Could you check a few things on this drawing? It's one solid part, dimensions in mm from its lowest x, y, z. Give positions to 0.01 mm unless a question says otherwise; leave off trailing zeros. Order: outer loops, then holes, each group sorted by start corner. A loop starts at its lowest first (then second) coordinate and runs counter-clockwise, first axis right, second up. Notation, with made-up numbers: (-7.5, 4.5) - (28.5, 4.5) arc R16 ccw to (28.5, 22.5) - close; hole circle Ø10 at (35, -30). An arc over 180 degrees is marked (long way). Return JSON: item names as keys, results as strings.
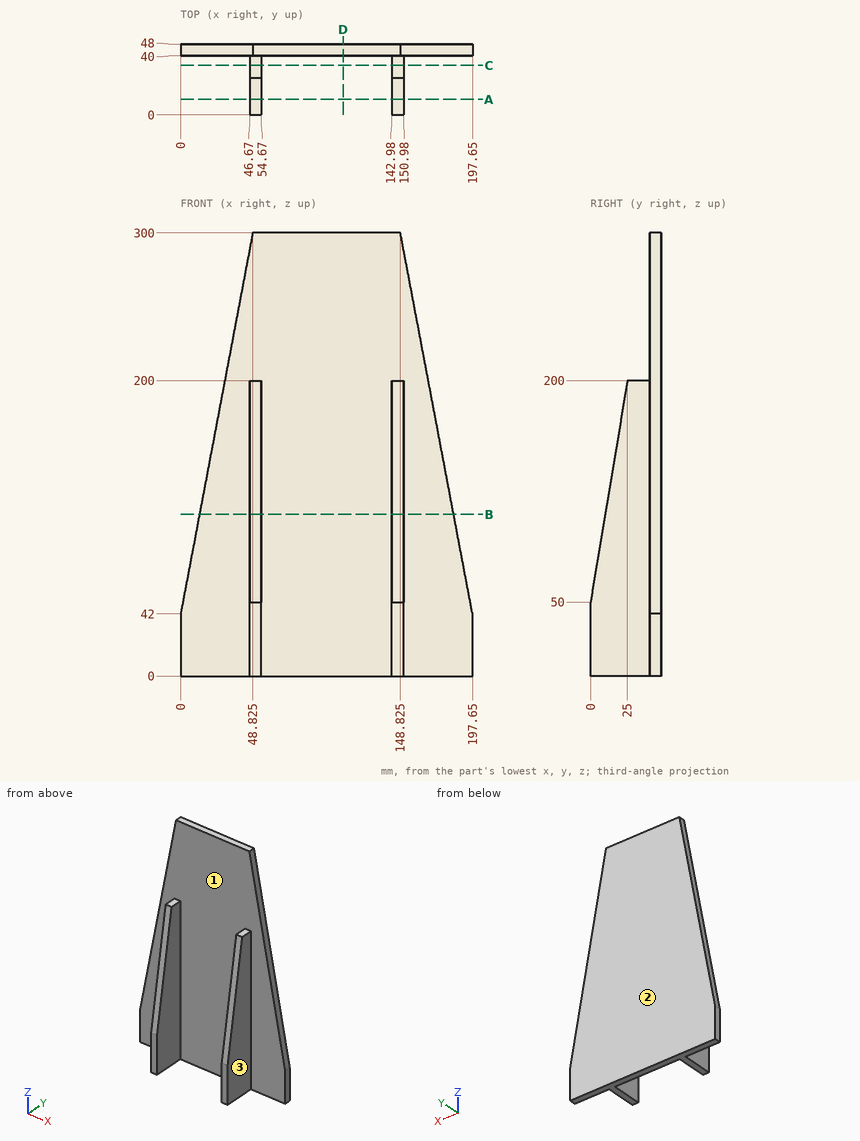
1. For pin 1 Ø1 at (x, z) = (82.5, 193.5) entering from -Y; pin 2 Ø12 at (y, z) = (20, 77.5) entering from +X; pin 3 Ø2.5 at (x, y) = (50, 31) entering from +Z, each with a flat end and sliding along its axis, tell me the tip position at first contact or that it passes through.
Checks:
{"pin 1": "y = 40", "pin 2": "x = 150.98", "pin 3": "z = 200"}
2. Suppose I cut it at B-B (z = 109.5). List the corners of the cut face in (x, y) for me.
Checks:
{"outline": "(12.77, 40) - (46.67, 40) - (46.67, 9.92) - (54.67, 9.92) - (54.67, 40) - (142.98, 40) - (142.98, 9.92) - (150.98, 9.92) - (150.98, 40) - (184.88, 40) - (184.88, 48) - (12.77, 48) - close"}
3. Suppose I cut it at C-C (y = 33.5). List the corners of the cut face in (x, z) for me, plus the area to 3 significant figures.
Checks:
{"outline": "(46.67, 0) - (54.67, 0) - (54.67, 200) - (46.67, 200) - close; (142.98, 0) - (150.98, 0) - (150.98, 200) - (142.98, 200) - close", "area": "3,200 mm^2"}
4. Thinking about a two-plate mould opening in X: for the marked faces 1, 2 and 3, which applies, +X half, -X half, draft (parallel to the pull), parting line (faces both ways), or undercut?
Checks:
{"face 1": "undercut", "face 2": "draft", "face 3": "+X half"}
5. Suppose I cut it at D-D (x = 110). List the corners of the cut face in (y, z) for me.
Checks:
{"outline": "(40, 0) - (48, 0) - (48, 300) - (40, 300) - close"}
6. If I drill on L1, parallel to X at y = 25.5, z = 180; L2, parallel to Y at x = 95.5, z = 96; L3, parallel to X at y = 43, z = 45, over which ranges is the centre line in solid material (lowest first)? Write a range as [from, to].
Checks:
{"L1": "[46.67, 54.67], [142.98, 150.98]", "L2": "[40, 48]", "L3": "[0.57, 197.08]"}
7. Suppose I cut it at A-A (y = 10.5). List the corners of the cut face in (x, z) for me, plus the area to 3 significant figures.
Checks:
{"outline": "(46.67, 0) - (54.67, 0) - (54.67, 113) - (46.67, 113) - close; (142.98, 0) - (150.98, 0) - (150.98, 113) - (142.98, 113) - close", "area": "1,810 mm^2"}
